```python
from build123d import *

# Parameters (mm, degrees)
BOSS_EXTRUDE1_DEPTH         = 10
CUT_EXTRUDE1_DEPTH          = 67.219332525
CUT_EXTRUDE2_DEPTH          = 2
M3_TAPPED_HOLE2_D           = 2.5
M3_TAPPED_HOLE2_DEPTH       = 9
M3_TAPPED_HOLE2_CSINK_D     = 3.05
M3_TAPPED_HOLE2_CSINK_ANGLE = 100
M3_TAPPED_HOLE2_TIP         = 0.751075774
SKETCH7_R                   = 2.5
CUT_EXTRUDE3_DEPTH          = 44.185645763
SKETCH8_R                   = 4
CUT_EXTRUDE4_DEPTH          = 53.191953403
CHAMFER1_SIZE               = 1
CUT_EXTRUDE5_REACH          = 54.192
CUT_EXTRUDE5_END_RADIUS     = 7
SKETCH11_R                  = 1.6
M4_TAPPED_HOLE1_REACH       = 68.219
M4_TAPPED_HOLE1_BORE_R      = 1.65
CUT_EXTRUDE6_REACH          = 68.219
CUT_EXTRUDE6_END_RADIUS     = 2.5
SKETCH14_R                  = 1.25


# Read off the part's stored shape, not the designer's step: Hole1
with BuildPart() as part:
    # Sketch1 → Boss-Extrude1 (new, symmetric)
    with BuildSketch(Plane.XY):
        Polygon((0, 0), (-19, 0), (-19, 32), (9, 32), (21, -6), (21, -30), (0, -30), align=None)
    extrude(amount=BOSS_EXTRUDE1_DEPTH, both=True)

    # Sketch2 → Cut-Extrude1 (cut, through all)
    with BuildSketch(Plane(origin=(0, 32, 0), x_dir=(1, 0, 0), z_dir=(0, 1, 0))):
        with BuildLine():
            ThreePointArc((-2.291796068, 2), (-10.010587075, 6.926666858), (-16, 0))
            Line((-16, 0), (-2, 0))
            ThreePointArc((-2, 0), (-2.073333142, 1.010587075), (-2.291796068, 2))
        make_face()
        with BuildLine():
            Line((-2, 0), (-16, 0))
            ThreePointArc((-16, 0), (-10.010587075, -6.926666858), (-2.291796068, -2))
            ThreePointArc((-2.291796068, -2), (-2.073333142, -1.010587075), (-2, 0))
        make_face()
    extrude(amount=-CUT_EXTRUDE1_DEPTH, mode=Mode.SUBTRACT)

    # Sketch2<3> → Cut-Extrude2 (cut)
    with BuildSketch(Plane(origin=(0, 32, 0), x_dir=(1, 0, 0), z_dir=(0, 1, 0))):
        with BuildLine():
            ThreePointArc((5, 2), (3.585786438, 1.414213562), (3, 0))
            Line((3, 0), (7, 0))
            ThreePointArc((7, 0), (6.414213562, 1.414213562), (5, 2))
        make_face()
        with BuildLine():
            Line((7, 0), (3, 0))
            ThreePointArc((3, 0), (3.585786438, -1.414213562), (5, -2))
            ThreePointArc((5, -2), (6.414213562, -1.414213562), (7, 0))
        make_face()
        with BuildLine():
            ThreePointArc((-2.291796068, 2), (-2.073333142, 1.010587075), (-2, 0))
            Line((-2, 0), (3, 0))
            ThreePointArc((3, 0), (3.585786438, 1.414213562), (5, 2))
            Line((5, 2), (-2.291796068, 2))
        make_face()
        with BuildLine():
            Line((3, 0), (-2, 0))
            ThreePointArc((-2, 0), (-2.073333142, -1.010587075), (-2.291796068, -2))
            Line((-2.291796068, -2), (5, -2))
            ThreePointArc((5, -2), (3.585786438, -1.414213562), (3, 0))
        make_face()
    extrude(amount=-CUT_EXTRUDE2_DEPTH, mode=Mode.SUBTRACT)

    # M3 Tapped Hole2
    with Locations(Plane(origin=(0, 32, 0), x_dir=(1, 0, 0), z_dir=(0, 1, 0))):
        with Locations((-16, 7), (-16, -7), (5, 7), (5, -7)):
            CounterSinkHole(M3_TAPPED_HOLE2_D / 2, M3_TAPPED_HOLE2_CSINK_D / 2, depth=M3_TAPPED_HOLE2_DEPTH, counter_sink_angle=M3_TAPPED_HOLE2_CSINK_ANGLE)
            with Locations((0, 0, -(M3_TAPPED_HOLE2_DEPTH + M3_TAPPED_HOLE2_TIP / 2))):  # 118° drill point
                Cone(0, M3_TAPPED_HOLE2_D / 2, M3_TAPPED_HOLE2_TIP, mode=Mode.SUBTRACT)

    # Sketch7 → Cut-Extrude3 (cut, through all)
    with BuildSketch(Plane.XY.offset(10)):
        with Locations((13, -10)):
            Circle(SKETCH7_R)
    extrude(amount=-CUT_EXTRUDE3_DEPTH, mode=Mode.SUBTRACT)

    # Sketch8 → Cut-Extrude4 (cut, through all)
    with BuildSketch(Plane(origin=(21, 0, 0), x_dir=(0, 0, -1), z_dir=(1, 0, 0))):
        with Locations(Location((0, -20, 0), (0, 0, 90))):
            Circle(SKETCH8_R)
    extrude(amount=-CUT_EXTRUDE4_DEPTH, mode=Mode.SUBTRACT)

    # Chamfer1
    chamfer1_edges = [part.edges().sort_by_distance(p)[0] for p in [
        (21, -24, 0),
    ]]
    chamfer(chamfer1_edges, length=CHAMFER1_SIZE)

    # Hole1 outline → Hole1 (revolve, cut)
    with BuildSketch(Plane(origin=(5, 0, 0), x_dir=(1, 0, 0), z_dir=(0, 0, 1))):
        Polygon((1.25, 2), (2, 2), (2, 32), (0, 32), (0, -16.200413917), (1.25, -16.200413917), align=None)
    revolve(axis=Axis((5, 0, 0), (0, 1, 0)), mode=Mode.SUBTRACT)

    # Cut-Extrude5: up to this cylinder (the profile starts outside it)
    cut_extrude5_end = Plane(origin=(-9, 15, 0), z_dir=(0, 1, 0)) * Cylinder(CUT_EXTRUDE5_END_RADIUS, 123.384, mode=Mode.PRIVATE)
    # Sketch11 → Cut-Extrude5 (cut, up to the surface)
    with BuildSketch(Plane.ZY.offset(19), mode=Mode.PRIVATE) as cut_extrude5_sk1:
        with Locations(Location((-3, 15, 0), (0, 0, 270))):
            Circle(SKETCH11_R)
    cut_extrude5_tool1 = extrude(cut_extrude5_sk1.sketch, amount=-CUT_EXTRUDE5_REACH, mode=Mode.PRIVATE) - cut_extrude5_end
    add(cut_extrude5_tool1.solids().sort_by_distance((-19, 15, -3))[0], mode=Mode.SUBTRACT)
    # Sketch11 → Cut-Extrude5 (cut, up to the surface)
    with BuildSketch(Plane.ZY.offset(19), mode=Mode.PRIVATE) as cut_extrude5_sk2:
        with Locations(Location((3, 15, 0), (0, 0, 270))):
            Circle(SKETCH11_R)
    cut_extrude5_tool2 = extrude(cut_extrude5_sk2.sketch, amount=-CUT_EXTRUDE5_REACH, mode=Mode.PRIVATE) - cut_extrude5_end
    add(cut_extrude5_tool2.solids().sort_by_distance((-19, 15, 3))[0], mode=Mode.SUBTRACT)

    # M4 Tapped Hole1 bore → M4 Tapped Hole1 (cut, up to next)
    with BuildSketch(Plane(origin=(0, -30, 0), x_dir=(-1, 0, 0), z_dir=(0, -1, 0)), mode=Mode.PRIVATE) as m4_tapped_hole1_sk1:
        with Locations((-13, 0)):
            Circle(M4_TAPPED_HOLE1_BORE_R)
    m4_tapped_hole1_tool1 = extrude(m4_tapped_hole1_sk1.sketch, amount=-M4_TAPPED_HOLE1_REACH, mode=Mode.PRIVATE) & part.part
    # M4 Tapped Hole1 bore → M4 Tapped Hole1 (cut, up to next)
    with BuildSketch(Plane(origin=(0, -30, 0), x_dir=(-1, 0, 0), z_dir=(0, -1, 0)), mode=Mode.PRIVATE) as m4_tapped_hole1_sk2:
        with Locations((-5, 0)):
            Circle(M4_TAPPED_HOLE1_BORE_R)
    m4_tapped_hole1_tool2 = extrude(m4_tapped_hole1_sk2.sketch, amount=-M4_TAPPED_HOLE1_REACH, mode=Mode.PRIVATE) & part.part
    add(m4_tapped_hole1_tool1.solids().sort_by_distance((13, -30, 0))[0], mode=Mode.SUBTRACT)
    add(m4_tapped_hole1_tool2.solids().sort_by_distance((5, -30, 0))[0], mode=Mode.SUBTRACT)

    # Cut-Extrude6: up to this cylinder (the profile starts outside it)
    cut_extrude6_end = Plane(origin=(13, -10, 0), z_dir=(0, 0, 1)) * Cylinder(CUT_EXTRUDE6_END_RADIUS, 142.438, mode=Mode.PRIVATE)
    # Sketch14 → Cut-Extrude6 (cut, up to the surface)
    with BuildSketch(Plane.XZ.offset(30), mode=Mode.PRIVATE) as cut_extrude6_sk1:
        with Locations((13, 0)):
            Circle(SKETCH14_R)
    cut_extrude6_tool1 = extrude(cut_extrude6_sk1.sketch, amount=-CUT_EXTRUDE6_REACH, mode=Mode.PRIVATE) - cut_extrude6_end
    add(cut_extrude6_tool1.solids().sort_by_distance((13, -30, 0))[0], mode=Mode.SUBTRACT)


solid = part.part
```
Geometry: final body of the model. Coordinates: model frame, mm. A direction names the side the tool comes from. Coordinates: 2 decimals unless noted, no trailing zeros. Loops run counter-clockwise (first coordinate to the right, second up) from the corner with the lowest first, then second, coordinate; pieces in that order, holes last. Notation, with made-up numbers: (81, 10) -> (98, 10) arc R24 cw to (98, 38) -> close; hole circle Ø8 at (68.5, 45). An arc over 180 degrees is marked (long way). Use a Markdown table: item, result. Add a question column.
(1) Mould query, pull axis Y, two halves, no side actions, for faces 3 (the conical face through (4.78, 22.38, 6.99)), 4 (the cylindrical face through (-17.196, 15.208, 4.586)), 5 (the cylindrical face through (5.99, 27.32, 7.76)). Classes: pulls with the +Y half, pulls with the -Y half, needs draft (parallel to the pull), parting line crosses it, or undercut.
(2) Section query A-A, the plane y = -20. Return loops of the section in (x, z).
(3) Section query D-D, the plane x = 13. Return loops of the section in (y, z).
(4) Pin query (flat end, axial travel): pin 1 Ø5.5 at (x, z) = (5, 0) entering from -Y; pin 2 Ø2 at (y, z) = (1.5, 1.5) entering from +X; pin 3 Ø2 at (x, z) = (-16, -7) entering from +Y; pin 4 Ø1 at (y, z) = (-2, 0.5) entering from +X. Return the tip coordinate at first contact, or that it passes through.
(5) Access query for faces 1 (the flat face through (1, 1, -10)), 2 (the cylindrical face through (-15.73, 27.32, 8.22)). Directions: +Z, -Z, +X, -X, +Y, -Y. A direction counts if a zero-diameter tool reaches every point of the face in a straight line with its end or side. Return the directions, or none.
(6) Section query C-C, the plane x = -6.5. Return loops of the section in (y, z), plus the area to 3 significant figures.
(7) Line query: line 1 along X through (y, z) = (-25.75, 0); line 2 along Z through (x, y) = (-16.15, 15); line 3 along Z through (x, y) = (-12.5, 29.5). Output: solid intervals per line, ascending.
(8) Section query B-B, the plane x = 2. Return loops of the section in (y, z), plus the area to 3 significant figures.
Answer:
| question | item | result |
|---|---|---|
| 1 | face 3 | pulls with the +Y half |
| 1 | face 4 | undercut |
| 1 | face 5 | needs draft |
| 2 | outline | (0, -10) -> (21, -10) -> (21, -5) -> (20, -4) -> (0, -4) -> close; (0, 4) -> (20, 4) -> (21, 5) -> (21, 10) -> (0, 10) -> close |
| 3 | outline | (-30, -10) -> (-12.5, -10) -> (-12.5, -1.25) -> (-16.2, -1.25) arc R4 cw to (-23.64, -1.65) -> (-30, -1.65) -> close; (-30, 1.65) -> (-23.64, 1.65) arc R4 cw to (-16.2, 1.25) -> (-12.5, 1.25) -> (-12.5, 10) -> (-30, 10) -> close; (-7.5, -10) -> (19.33, -10) -> (19.33, 10) -> (-7.5, 10) -> close |
| 4 | pin 1 | stops at y = -30 |
| 4 | pin 2 | stops at x = 18.95 |
| 4 | pin 3 | stops at y = 22.85 |
| 4 | pin 4 | stops at x = 19.89 |
| 5 | face 1 | -Z, +X, -X, +Y, -Y |
| 5 | face 2 | +Y |
| 6 | outline | (0, -10) -> (32, -10) -> (32, -6.54) -> (0, -6.54) -> close; (0, 6.54) -> (32, 6.54) -> (32, 10) -> (0, 10) -> close |
| 6 | area | 222 mm^2 |
| 7 | line 1 | x = 0 to 3.35, 6.65 to 11.35, 14.65 to 21 |
| 7 | line 2 | z = -10 to -4.6, -1.4 to 1.4, 4.6 to 10 |
| 7 | line 3 | z = -10 to -6.06, 6.06 to 10 |
| 8 | outline | (-30, -10) -> (32, -10) -> (32, -2) -> (30, -2) -> (30, 2) -> (32, 2) -> (32, 10) -> (-30, 10) -> close; hole circle Ø8 at (-20, 0) |
| 8 | area | 1,180 mm^2 |
